Part print with two shaded views. Sizes in mm from the minimum x, y, z corner. Round coordinates to 2 decimals unless told otherwise and drop trailing zeros. Loops run counter-clockwise (first coordinate to the right, second up) from the corner with the lowest first, then second, coordinate; pieces in that order, holes last.
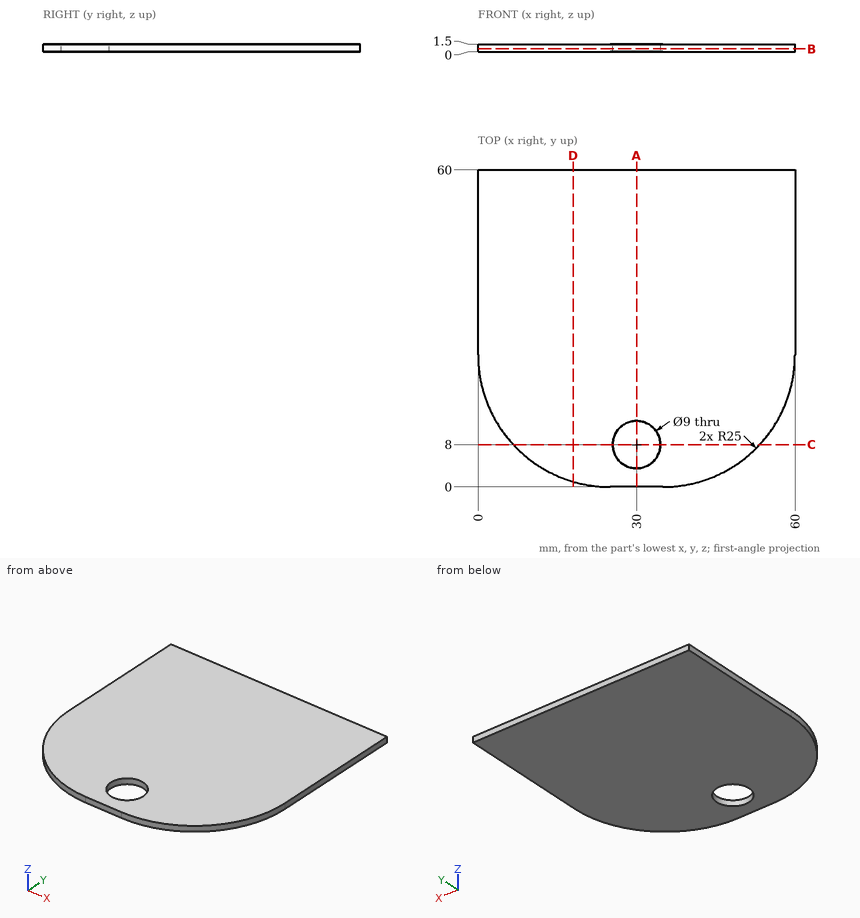
Item 1: Cut at A-A (x = 30). List the corners of the cut face in (y, z).
Verdict:
outline: (0, 0) - (3.5, 0) - (3.5, 1.5) - (0, 1.5) - close; (12.5, 0) - (60, 0) - (60, 1.5) - (12.5, 1.5) - close
Item 2: Wall check: L1, parallel to Y at x = 30, z = 1.2; L2, parallel to X at y = 8, z = 0.6; L3, parallel to Y at x = 24.5, z = 1.4 (3 decimals). Give the ranges that are in metal, low to high.
Verdict:
L1: y = 0 to 3.5, 12.5 to 60
L2: x = 6.67 to 25.5, 34.5 to 53.33
L3: y = 0.005 to 60
Item 3: Cut at B-B (z = 0.6). List the corners of the cut face in (x, y).
Verdict:
outline: (0, 25) arc R25 ccw to (25, 0) - (35, 0) arc R25 ccw to (60, 25) - (60, 60) - (0, 60) - close; hole circle Ø9 at (30, 8)
Item 4: Cut at D-D (x = 18). List the corners of the cut face in (y, z), plus the area to 3 significant figures.
Verdict:
outline: (1, 0) - (60, 0) - (60, 1.5) - (1, 1.5) - close
area: 88.5 mm2
Item 5: Cut at C-C (y = 8). List the corners of the cut face in (x, z), plus the area to 3 significant figures.
Verdict:
outline: (6.67, 0) - (25.5, 0) - (25.5, 1.5) - (6.67, 1.5) - close; (34.5, 0) - (53.33, 0) - (53.33, 1.5) - (34.5, 1.5) - close
area: 56.5 mm2
